Source: CAD feature listing. Evaluate the final solid. Frame: model axes, mm. Coordinates: 2 decimals unless noted, no trailing zeros. Write item = value, one per line. Start each with the question number.
Item 1: Contact query for a flat-ended pin moving along its axis: pin 1 (3 mm diameter, centred on x = -46.62, z = -18.3, fed in from -Y). Output: stop coordinate, or through.
Item 2: Section query A-A (y = 3.15). Count the separate pieces of the cut face and the enclosed holes in it, then the cut area to 3 significant figures.
Item 3: Ray query, line 1 along Z through (x, y) = (127.5, 3.85); line 2 along X through (y, z) = (4.7, -10); line 3 along X through (y, z) = (2.2, 131.5). Return the intervals inside material, ascending. Write a range as [from, to].
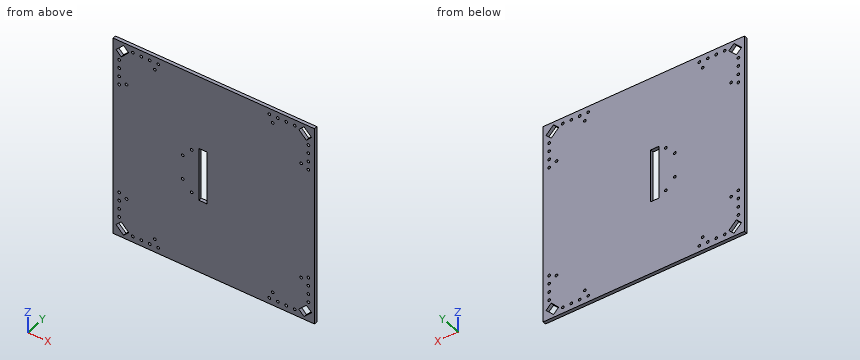
```python
from build123d import *

# Parameters (mm, degrees)
SKETCH1_W               = 301.625
SKETCH1_H               = 301.625
BOSS_EXTRUDE1_DEPTH     = 5
CUT_EXTRUDE1_DEPTH      = 10
SKETCH4_W               = 12.5
SKETCH4_H               = 80
CUT_EXTRUDE3_DEPTH      = 214.33968293
SKETCH5_R               = 2
CUT_EXTRUDE4_DEPTH      = 10
MIRROR2_COPY_1_SKETCH_R = 2
MIRROR2_COPY_1_DEPTH    = 10
MIRROR3_COPY_1_SKETCH_R = 2
MIRROR3_COPY_1_DEPTH    = 10
MIRROR3_COPY_2_SKETCH_R = 2
MIRROR3_COPY_2_DEPTH    = 10
MIRROR3_COPY_3_SKETCH_R = 2
MIRROR3_COPY_3_DEPTH    = 10
SKETCH6_R               = 2
CUT_EXTRUDE5_DEPTH      = 214.33968293


with BuildPart() as part:
    # Sketch1 → Boss-Extrude1 (new body)
    with BuildSketch(Plane(origin=(0, 0, 0), x_dir=(1, 0, 0), z_dir=(0, 1, 0))):
        Rectangle(SKETCH1_W, SKETCH1_H)
    extrude(amount=BOSS_EXTRUDE1_DEPTH)

    # Sketch2 → Cut-Extrude1 (cut)
    with BuildSketch(Plane.XZ):
        Polygon((127.420616908, 138.734325407), (138.734325407, 127.420616908), (146.5125, 135.198791501), (135.198791501, 146.5125), align=None)
        Polygon((146.5125, -135.198791501), (138.734325407, -127.420616908), (127.420616908, -138.734325407), (135.198791501, -146.5125), align=None)
        Polygon((-135.198791501, -146.5125), (-127.420616908, -138.734325407), (-138.734325407, -127.420616908), (-146.5125, -135.198791501), align=None)
        Polygon((-146.5125, 135.198791501), (-138.734325407, 127.420616908), (-127.420616908, 138.734325407), (-135.198791501, 146.5125), align=None)
    extrude(amount=-CUT_EXTRUDE1_DEPTH, mode=Mode.SUBTRACT)

    # Sketch4 → Cut-Extrude3 (cut, through all)
    with BuildSketch(Plane(origin=(0, 5, 0), x_dir=(1, 0, 0), z_dir=(0, 1, 0))):
        with Locations((-16.25, 0)):
            Rectangle(SKETCH4_W, SKETCH4_H)
    extrude(amount=-CUT_EXTRUDE3_DEPTH, mode=Mode.SUBTRACT)

    # Sketch5 → Cut-Extrude4 (cut)
    with BuildSketch(Plane(origin=(0, 5, 0), x_dir=(1, 0, 0), z_dir=(0, 1, 0))):
        with Locations(Location((-130.8125, 88.3125, 0), (0, 0, 270))):
            Circle(SKETCH5_R)
        with Locations(Location((-141.8125, 95.979166667, 0), (0, 0, 270))):
            Circle(SKETCH5_R)
        with Locations(Location((-141.8125, 83.3125, 0), (0, 0, 270))):
            Circle(SKETCH5_R)
        with Locations(Location((-141.8125, 108.645833333, 0), (0, 0, 270))):
            Circle(SKETCH5_R)
        with Locations(Location((-141.8125, 121.3125, 0), (0, 0, 270))):
            Circle(SKETCH5_R)
    cut_extrude4 = extrude(amount=-CUT_EXTRUDE4_DEPTH, mode=Mode.SUBTRACT)

    # Mirror1: Cut-Extrude4 across plane
    add(cut_extrude4.mirror(Plane(origin=(0, 0, 0), x_dir=(0.7071067811865476, 0, 0.7071067811865476), z_dir=(-0.7071067811865477, 0, 0.7071067811865475))), mode=Mode.SUBTRACT)

    # Mirror2: Cut-Extrude4 across plane
    add(cut_extrude4.mirror(Plane.XY), mode=Mode.SUBTRACT)

    # Mirror2 copy 1 sketch → Mirror2 copy 1 (cut)
    with BuildSketch(Plane(origin=(0, 5, 0), x_dir=(0, 0, -1), z_dir=(0, 1, 0))):
        with Locations(Location((-130.8125, 88.3125, 0), (0, 0, 270))):
            Circle(MIRROR2_COPY_1_SKETCH_R)
        with Locations(Location((-141.8125, 95.979166667, 0), (0, 0, 270))):
            Circle(MIRROR2_COPY_1_SKETCH_R)
        with Locations(Location((-141.8125, 83.3125, 0), (0, 0, 270))):
            Circle(MIRROR2_COPY_1_SKETCH_R)
        with Locations(Location((-141.8125, 108.645833333, 0), (0, 0, 270))):
            Circle(MIRROR2_COPY_1_SKETCH_R)
        with Locations(Location((-141.8125, 121.3125, 0), (0, 0, 270))):
            Circle(MIRROR2_COPY_1_SKETCH_R)
    extrude(amount=-MIRROR2_COPY_1_DEPTH, mode=Mode.SUBTRACT)

    # Mirror3: Cut-Extrude4 across plane
    add(cut_extrude4.mirror(Plane(origin=(0, 0, 0), x_dir=(0, 0, 1), z_dir=(1, 0, 0))), mode=Mode.SUBTRACT)

    # Mirror3 copy 1 sketch → Mirror3 copy 1 (cut)
    with BuildSketch(Plane.ZX.offset(5)):
        with Locations(Location((-130.8125, 88.3125, 0), (0, 0, 270))):
            Circle(MIRROR3_COPY_1_SKETCH_R)
        with Locations(Location((-141.8125, 95.979166667, 0), (0, 0, 270))):
            Circle(MIRROR3_COPY_1_SKETCH_R)
        with Locations(Location((-141.8125, 83.3125, 0), (0, 0, 270))):
            Circle(MIRROR3_COPY_1_SKETCH_R)
        with Locations(Location((-141.8125, 108.645833333, 0), (0, 0, 270))):
            Circle(MIRROR3_COPY_1_SKETCH_R)
        with Locations(Location((-141.8125, 121.3125, 0), (0, 0, 270))):
            Circle(MIRROR3_COPY_1_SKETCH_R)
    extrude(amount=-MIRROR3_COPY_1_DEPTH, mode=Mode.SUBTRACT)

    # Mirror3 copy 2 sketch → Mirror3 copy 2 (cut)
    with BuildSketch(Plane(origin=(0, 5, 0), x_dir=(-1, 0, 0), z_dir=(0, 1, 0))):
        with Locations(Location((-130.8125, 88.3125, 0), (0, 0, 270))):
            Circle(MIRROR3_COPY_2_SKETCH_R)
        with Locations(Location((-141.8125, 95.979166667, 0), (0, 0, 270))):
            Circle(MIRROR3_COPY_2_SKETCH_R)
        with Locations(Location((-141.8125, 83.3125, 0), (0, 0, 270))):
            Circle(MIRROR3_COPY_2_SKETCH_R)
        with Locations(Location((-141.8125, 108.645833333, 0), (0, 0, 270))):
            Circle(MIRROR3_COPY_2_SKETCH_R)
        with Locations(Location((-141.8125, 121.3125, 0), (0, 0, 270))):
            Circle(MIRROR3_COPY_2_SKETCH_R)
    extrude(amount=-MIRROR3_COPY_2_DEPTH, mode=Mode.SUBTRACT)

    # Mirror3 copy 3 sketch → Mirror3 copy 3 (cut)
    with BuildSketch(Plane(origin=(0, 5, 0), x_dir=(0, 0, -1), z_dir=(0, 1, 0))):
        with Locations((-130.8125, -88.3125)):
            Circle(MIRROR3_COPY_3_SKETCH_R)
        with Locations((-141.8125, -95.979166667)):
            Circle(MIRROR3_COPY_3_SKETCH_R)
        with Locations((-141.8125, -83.3125)):
            Circle(MIRROR3_COPY_3_SKETCH_R)
        with Locations((-141.8125, -108.645833333)):
            Circle(MIRROR3_COPY_3_SKETCH_R)
        with Locations((-141.8125, -121.3125)):
            Circle(MIRROR3_COPY_3_SKETCH_R)
    extrude(amount=-MIRROR3_COPY_3_DEPTH, mode=Mode.SUBTRACT)

    # Sketch6 → Cut-Extrude5 (cut, through all)
    with BuildSketch(Plane(origin=(0, 5, 0), x_dir=(1, 0, 0), z_dir=(0, 1, 0))):
        with Locations(Location((-33.1225, -32.7, 0), (0, 0, 270))):
            Circle(SKETCH6_R)
        with Locations(Location((-46.6225, -18.3, 0), (0, 0, 270))):
            Circle(SKETCH6_R)
        with Locations(Location((-46.6225, 18.3, 0), (0, 0, 270))):
            Circle(SKETCH6_R)
        with Locations(Location((-33.1225, 32.7, 0), (0, 0, 270))):
            Circle(SKETCH6_R)
    extrude(amount=-CUT_EXTRUDE5_DEPTH, mode=Mode.SUBTRACT)


solid = part.part
```
Computed:
q1.pin_1 = through
q2.separate_pieces = 1
q2.enclosed_holes = 49
q2.area = 88,700 mm^2
q3.line_1 = [-150.81, -138.81], [-138.65, 138.65], [138.81, 150.81]
q3.line_2 = [-150.81, -22.5], [-10, 150.81]
q3.line_3 = [-150.81, -142.81], [-134.65, -90.19], [-86.43, 86.43], [90.19, 134.65], [142.81, 150.81]
